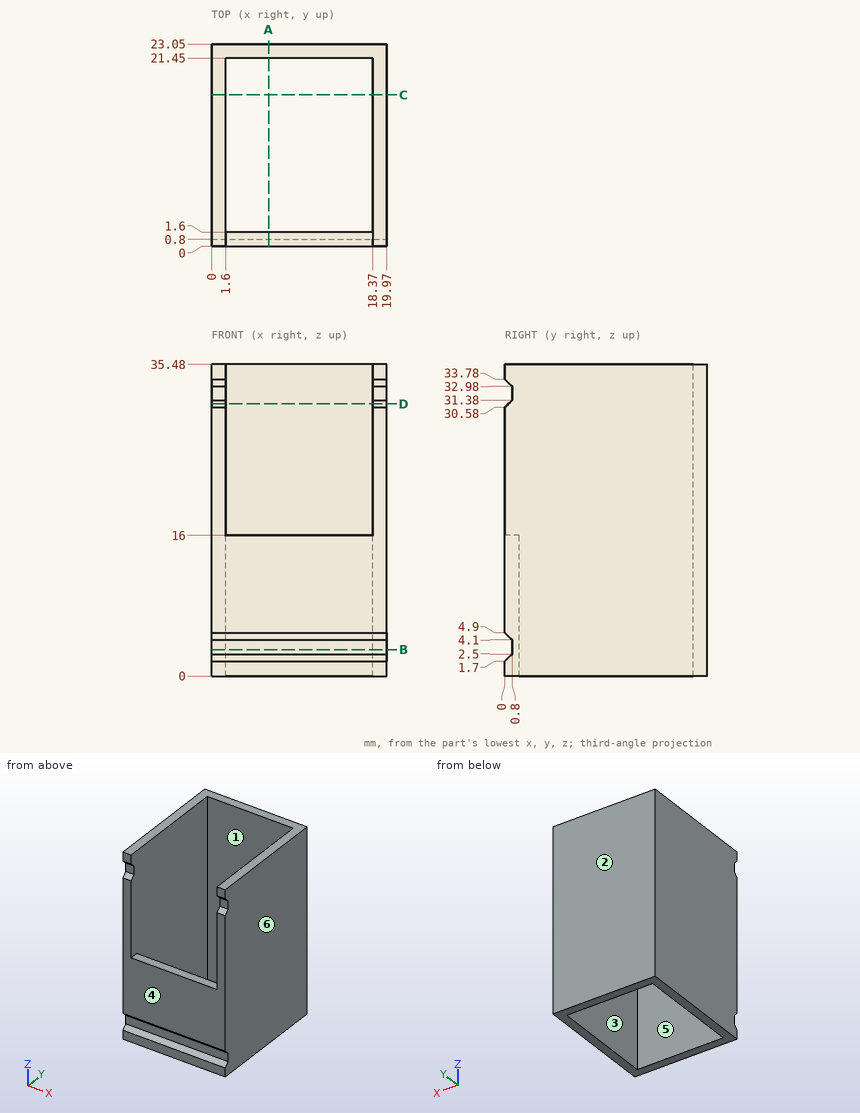
Geometry check sheet. Reference: drawing and pictorial views, mm from the part's lowest x, y, z. A direction names the side the tool comes from. Round coordinates to 2 decimals unless told otherwise and drop trailing zeros. Order: outer loops, then holes, each group sorted by start corner. A loop starts at its lowest first (then second) coordinate and runs counter-clockwise, first axis right, second up. Notation, with made-up numbers: M -25,-37.5 L 22,-37.5 A14 cw 22,-16.5 Z; hole C -23.75,1.25 d6. An arc over 180 degrees is marked long. One line per item, written item: value. Start each with the question number.
1. Access from +Z, -Z, +X, -X, +Y, -Y to the whole of each face (thin tool, end or side, straight path). Record for the marked faces 5 and 6.
2. Release check for a two-part mould opening along Y. For the marked faces 1, 2, 3 and 4 record: released by +Y, released by -Y, zero draft, split by the parting line, or undercut.
3. Section check D-D on z = 31. Enter the section's corners in (x, y).
4. Section check C-C on y = 17.25. Enter the section's corners in (x, z), and give its area (3 significant figures).
5. Gauge pin test, flat ends, axial feed: P1, Ø0.5, axis at x = 0.5, z = 32, coming from the -Y side; P2, Ø8, axis at y = 16, z = 18.5, coming from the -X side; P3, Ø1.3, axis at x = 19, z = 32.5, coming from the -Y side; P4, Ø1.3, axis at x = 11.5, y = 1, coming from the +Z side. Record the tip position at first contact, or that the pin passes through.
6. Section check A-A on x = 6.5. Enter the section's corners in (y, z).
7. Section check B-B on z = 3. Enter the section's corners in (x, y).
8. Scan lines: line 1 along Y through (x, z) = (3.5, 13); line 2 along X through (y, z) = (13, 11.5); line 3 along Y through (x, z) = (8, 28.5). Record each from-to range of solid material in increasing order.
Results found:
1. face 5: +Z, -Z
1. face 6: +Z, -Z, +X, +Y, -Y
2. face 1: undercut
2. face 2: released by +Y
2. face 3: undercut
2. face 4: released by -Y
3. outline: M 0,0.42 L 1.6,0.42 L 1.6,21.45 L 18.37,21.45 L 18.37,0.42 L 19.97,0.42 L 19.97,23.05 L 0,23.05 Z
4. outline: M 0,0 L 1.6,0 L 1.6,35.48 L 0,35.48 Z; M 18.37,0 L 19.97,0 L 19.97,35.48 L 18.37,35.48 Z
4. area: 114 mm^2
5. P1: y = 0.8
5. P2: x = 0
5. P3: y = 0.63
5. P4: z = 16
6. outline: M 0,0 L 1.6,0 L 1.6,16 L 0,16 L 0,4.9 L 0.8,4.1 L 0.8,2.5 L 0,1.7 Z; M 21.45,0 L 23.05,0 L 23.05,35.48 L 21.45,35.48 Z
7. outline: M 0,0.8 L 19.97,0.8 L 19.97,23.05 L 0,23.05 Z; hole M 1.6,1.6 L 18.37,1.6 L 18.37,21.45 L 1.6,21.45 Z
8. line 1: 0 to 1.6, 21.45 to 23.05
8. line 2: 0 to 1.6, 18.37 to 19.97
8. line 3: 21.45 to 23.05
